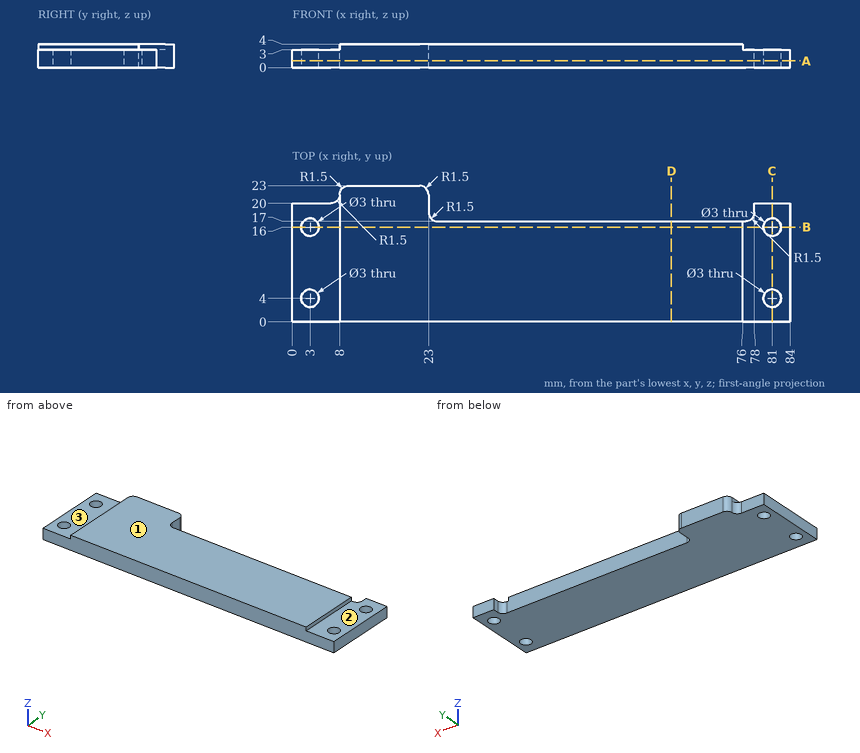
Geometry check sheet. Reference: drawing and pictorial views, mm from the part's lowest x, y, z. A direction names the side the tool comes from. Round coordinates to 2 decimals unless told otherwise and drop trailing zeros. Loops run counter-clockwise (first coordinate to the right, second up) from the corner with the lowest first, then second, coordinate; pieces in that order, holes last. Notation, with made-up numbers: M 55.5,82.25 L 78.5,82.25 A26 ccw 78.5,112.25 Z; hole C -31.5,47.5 d5. An arc over 180 degrees is marked long. One line per item, written item: value.
(1) Sectioned sample at A-A, the plane z = 1.15. Count the separate pieces of the cut face and the enclosed holes in it, then the cut area to 3 significant figures.
Computed values:
separate pieces: 1
enclosed holes: 4
area: 1,530 mm^2
(2) Thickness scan on line 1 (Y direction, x = 3, z = 0.8); line 2 (X direction, y = 16, z = 2.3); line 3 (X direction, y = 5.25, z = 2.2). Record the ranges inside material, lowest first.
Computed values:
line 1: y = 0 to 2.5, 5.5 to 14.5, 17.5 to 20
line 2: x = 0 to 1.5, 4.5 to 79.5, 82.5 to 84
line 3: x = 0 to 2.17, 3.83 to 80.17, 81.83 to 84
(3) Sectioned sample at C-C, the plane x = 81. Record the cut outline in (y, z).
Computed values:
outline: M 0,0 L 2.5,0 L 2.5,3 L 0,3 Z; M 5.5,0 L 14.5,0 L 14.5,3 L 5.5,3 Z; M 17.5,0 L 20,0 L 20,3 L 17.5,3 Z
(4) Sectioned sample at B-B, the plane y = 16. Record the cut outline in (x, z), then the cut area to 3 significant figures.
Computed values:
outline: M 0,0 L 1.5,0 L 1.5,3 L 0,3 Z; M 4.5,0 L 79.5,0 L 79.5,3 L 76,3 L 76,4 L 8,4 L 8,3 L 4.5,3 Z; M 82.5,0 L 84,0 L 84,3 L 82.5,3 Z
area: 302 mm^2
(5) Depth check by flat-ended pin: pin 1 Ø2.5 at (x, y) = (78.5, 14.5) entering from +Z; pin 2 Ø0.9 at (x, z) = (1.5, 2) entering from +Y; pin 3 Ø1.8 at (x, y) = (3, 4) entering from +Z; pin 4 Ø0.5 at (y, z) = (7.5, 3.5) entering from +X. Enter the tip coordinate at first touch or a pass-through.
Computed values:
pin 1: stops at z = 3
pin 2: stops at y = 20
pin 3: passes through
pin 4: stops at x = 76
(6) Access from +Z, -Z, +X, -X, +Y, -Y to the whole of each face (thin tool, end or side, straight path). Record for the marked faces 1, 2 and 3.
Computed values:
face 1: +Z, +X, -X, +Y, -Y
face 2: +Z, +X, +Y, -Y
face 3: +Z, -X, +Y, -Y
(7) Sectioned sample at D-D, the plane x = 64. Record the cut outline in (y, z), then the cut area to 3 significant figures.
Computed values:
outline: M 0,0 L 17,0 L 17,4 L 0,4 Z
area: 68.0 mm^2
